```python
from build123d import *

# Parameters (mm, degrees)
F1_DEPTH = 38.1


with BuildPart() as f1:
    # F0 (on Front) → F1 (new body)
    with BuildSketch(Plane.XZ):
        with BuildLine():
            Line((-63.5, -9.525), (63.5, -9.525))
            Line((63.5, -9.525), (63.5, 9.525))
            ThreePointArc((63.5, 9.525), (52.401686, 15.986353), (40.653953, 21.174071))
            Line((40.653953, 21.174071), (40.653953, 13.069536))
            ThreePointArc((40.653953, 13.069536), (37.901271, 5.160722), (35.878753, 13.286977))
            Line((35.878753, 13.286977), (35.878753, 22.853614))
            ThreePointArc((35.878753, 22.853614), (0, 28.575), (-35.878753, 22.853614))
            Line((-35.878753, 22.853614), (-35.878753, 13.286977))
            ThreePointArc((-35.878753, 13.286977), (-37.901271, 5.160722), (-40.653953, 13.069536))
            Line((-40.653953, 13.069536), (-40.653953, 21.174071))
            ThreePointArc((-40.653953, 21.174071), (-52.401686, 15.986353), (-63.5, 9.525))
            Line((-63.5, 9.525), (-63.5, -9.525))
        make_face()
    extrude(amount=-F1_DEPTH)


solid = f1.part
```
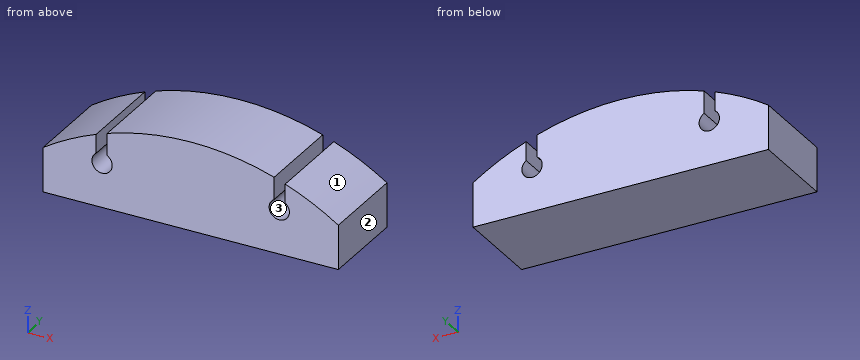
Check sheet for the modelled part. Datum: model origin and axes. Units: mm. Face numbers are marked on the shaded views. Give positions to 0.01 mm unless a question says otherwise; leave off trailing zeros. Write each loop counter-clockwise with the first axis right and the second up, starting at its lowest first coordinate (ties: lowest second). Pieces come first, ordered by that corner, then holes.
Item 1: Cross-section at B-B (x = 38.1). Enter the section's corners in (y, z) (3 decimals), and give its area (3 significant figures).
Item 2: Draft check along Z on the marked faces 1, 2 and 3. Enter one of: released by +Z, released by -Z, zero draft, split by the parting line, or undercut.
Item 3: Scan lines: L1, parallel to X at y = 29.5, z = 17; L2, parallel to X at y = 25, z = 18; L3, parallel to Z at x = -38, y = 16 (3 decimals). Record each from-to range of solid material in increasing order.
Item 4: Gauge pin test, flat ends, axial feed: pin 1 (4 mm diameter, centred on x = -15, y = 31, fed in from +Z); pin 2 (5 mm diameter, centred on y = 23, z = 20, fed in from +X); pin 3 (5 mm diameter, centred on x = -25, y = 10.5, fed in from +Z). Record the tip position at first contact, or that the pin passes through.
Item 5: Cross-section at A-A (y = 27). Enter the section's corners in (x, z) (3 decimals), and give its area (3 significant figures).
Report:
1. outline: (0, -9.525) - (38.1, -9.525) - (38.1, 5.156) - (0, 5.156) - close
1. area: 559 mm2
2. face 1: released by +Z
2. face 2: zero draft
2. face 3: undercut
3. L1: x = -50.36 to -40.65, -35.88 to 35.88, 40.65 to 50.36
3. L2: x = -48.25 to -40.65, -35.88 to 35.88, 40.65 to 48.25
3. L3: z = -9.525 to 5.157
4. pin 1: stops at z = 27.84
4. pin 2: stops at x = 49.32
4. pin 3: stops at z = 26.36
5. outline: (-63.5, -9.525) - (63.5, -9.525) - (63.5, 9.525) arc R115.358 ccw to (40.654, 21.174) - (40.654, 13.07) arc R4.369 cw (long way) to (35.879, 13.287) - (35.879, 22.854) arc R115.358 ccw to (-35.879, 22.854) - (-35.879, 13.287) arc R4.369 cw (long way) to (-40.654, 13.07) - (-40.654, 21.174) arc R115.358 ccw to (-63.5, 9.525) - close
5. area: 3,860 mm2
